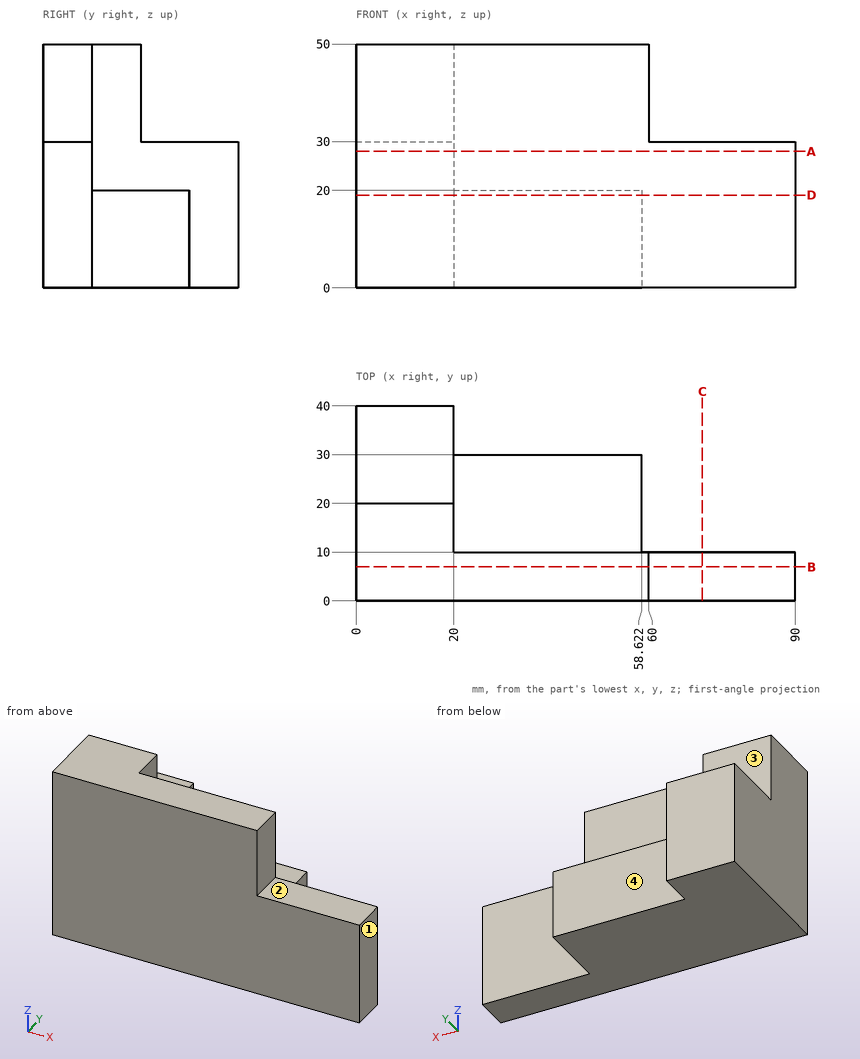
Here's the drawing with two shaded views (mm, measured from the low corner). I have some questions. A direction names the side the tool comes from. Coordinates: 2 decimals unless noted, no trailing zeros. Loops run counter-clockwise (first coordinate to the right, second up) from the corner with the lowest first, then second, coordinate; pieces in that order, holes last. Notation, with made-up numbers: (13.25, 11) -> (35.25, 11) arc R11 cw to (35.25, 30) -> close; hole circle Ø3 at (68, 18). An arc over 180 degrees is marked (long way). Answer as a JSON object with one key per item and string values.
1) For P1, Ø16, axis at y = 18.5, z = 5.5, coming from the +X side; P2, Ø22, axis at x = 44, z = 6.5, coming from the +Y side; P3, Ø1.5, axis at x = 59, z = 43.5, coming from the -Y side; P4, Ø5, axis at y = 5, z = 35.5, coming from the +X side, each with a flat end and sliding along its axis, tell me the tip position at first contact or that it passes through.
Results:
{"P1": "stops at x = 58.62", "P2": "stops at y = 30", "P3": "stops at y = 0", "P4": "stops at x = 60"}
2) Imagine slicing it at C-C (x = 71). Please give me the cut outline in (y, z), then the cut area to 3 significant figures.
Results:
{"outline": "(0, 0) -> (10, 0) -> (10, 30) -> (0, 30) -> close", "area": "300 mm^2"}
3) If I drill on line 1 (X direction, y = 5.5, z = 40); line 2 (X direction, y = 30.5, z = 18); line 3 (Y direction, x = 40.5, z = 13.5), over which ranges is the centre line in solid material (lowest first)?
Results:
{"line 1": "x = 0 to 60", "line 2": "x = 0 to 20", "line 3": "y = 0 to 30"}
4) Imagine slicing it at A-A (z = 28). Please give me the cut outline in (x, y).
Results:
{"outline": "(0, 0) -> (90, 0) -> (90, 10) -> (20, 10) -> (20, 40) -> (0, 40) -> close"}
5) For the marked faces 1, 2, 3 and 4, which set-ups out of +Z, -Z, +X, -X, +Y, -Y let a thin tool reach every point of the face, with its end or its side?
Results:
{"face 1": "+Z, -Z, +X, +Y, -Y", "face 2": "+Z, +X, +Y, -Y", "face 3": "+Z, +X, -X, +Y", "face 4": "+Z, -Z, +X, +Y"}
6) Imagine slicing it at D-D (z = 19). Please give me the cut outline in (x, y), then the cut area to 3 significant figures.
Results:
{"outline": "(0, 0) -> (90, 0) -> (90, 10) -> (58.62, 10) -> (58.62, 30) -> (20, 30) -> (20, 40) -> (0, 40) -> close", "area": "2,270 mm^2"}
7) Imagine slicing it at B-B (y = 7). Please give me the cut outline in (x, z).
Results:
{"outline": "(0, 0) -> (90, 0) -> (90, 30) -> (60, 30) -> (60, 50) -> (0, 50) -> close"}
